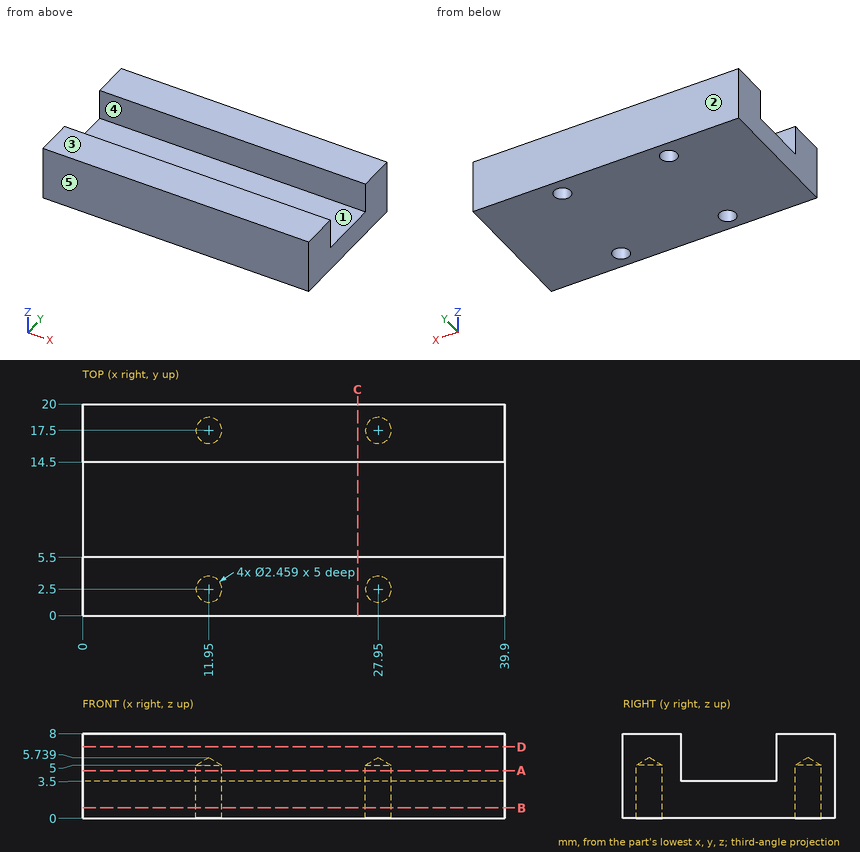
Study the drawing (mm; zero at the part's minimum x, y, z) and answer. A direction names the side the tool comes from. Coordinates: 2 decimals unless noted, no trailing zeros. Loops run counter-clockwise (first coordinate to the right, second up) from the corner with the lowest first, then second, coordinate; pieces in that order, holes last. Notation, with made-up numbers: M 33.5,70.25 L 78.5,70.25 A4 ccw 78.5,75.25 Z; hole C 40,5.5 d6. An arc over 180 degrees is marked long. Answer in a Markdown table with one row per item.
1) Find the intervals of material crossed by probe 1 along X at (y, z) = (17.5, 1.95); probe 2 along Y at (x, z) = (11.95, 2.45); probe 3 along Y at (x, z) = (27.95, 3.9), in increasing order.
Answers below:
| item | result |
|---|---|
| probe 1 | 0 to 10.72, 13.18 to 26.72, 29.18 to 39.9 |
| probe 2 | 0 to 1.27, 3.73 to 16.27, 18.73 to 20 |
| probe 3 | 0 to 1.27, 3.73 to 5.5, 14.5 to 16.27, 18.73 to 20 |
2) Find section D-D (z = 6.75). Determine the outline of the cut face in (x, y), then the cut area to 3 significant figures.
Answers below:
| item | result |
|---|---|
| outline | M 0,0 L 39.9,0 L 39.9,5.5 L 0,5.5 Z; M 0,14.5 L 39.9,14.5 L 39.9,20 L 0,20 Z |
| area | 439 mm^2 |
3) Find section A-A (z = 4.5). Determine the outline of the cut face in (x, y), then the cut area to 3 significant figures.
Answers below:
| item | result |
|---|---|
| outline | M 0,0 L 39.9,0 L 39.9,5.5 L 0,5.5 Z; M 0,14.5 L 39.9,14.5 L 39.9,20 L 0,20 Z; hole C 11.95,2.5 d2.46; hole C 11.95,17.5 d2.46; hole C 27.95,2.5 d2.46; hole C 27.95,17.5 d2.46 |
| area | 420 mm^2 |
4) Find section C-C (x = 26). Determine the outline of the cut face in (y, z).
Answers below:
| item | result |
|---|---|
| outline | M 0,0 L 20,0 L 20,8 L 14.5,8 L 14.5,3.5 L 5.5,3.5 L 5.5,8 L 0,8 Z |
5) Which of the six approach directions +Z, -Z, +X, -X, +Y, -Y give full straight-line access (tool end or side, diameter ignored) to the marked faces 4 and 5?
Answers below:
| item | result |
|---|---|
| face 4 | +Z, +X, -X |
| face 5 | +Z, -Z, +X, -X, -Y |
6) Determine the mould class of the marked faces 1, 2 and 3 for opening direction Y: released by +Y, released by -Y, zero draft, split by the parting line, or undercut.
Answers below:
| item | result |
|---|---|
| face 1 | undercut |
| face 2 | released by +Y |
| face 3 | zero draft |
7) Given pin 1 (2 mm diameter, centred on y = 13, z = 2.5, fed in from -X); pin 2 (2 mm diameter, centred on x = 27.95, y = 2.5, fed in from -Z), each flat-ended and moving along its own axis, determine where each tip first touches the part or whether it passes through.
Answers below:
| item | result |
|---|---|
| pin 1 | x = 0 |
| pin 2 | z = 5.14 |
8) Find section B-B (z = 1). Determine the outline of the cut face in (x, y).
Answers below:
| item | result |
|---|---|
| outline | M 0,0 L 39.9,0 L 39.9,20 L 0,20 Z; hole C 11.95,2.5 d2.46; hole C 11.95,17.5 d2.46; hole C 27.95,2.5 d2.46; hole C 27.95,17.5 d2.46 |
